Build history of the part. All positions in model axes, mm. Face numbers are marked on the shaded views. A direction names the side the tool comes from. Give positions to 0.01 mm unless a question says otherwise; leave off trailing zeros. Loops run counter-clockwise (first coordinate to the right, second up) from the corner with the lowest first, then second, coordinate; pieces in that order, holes last. Notation, with made-up numbers: M -5,-14 L 35,-14 A17 ccw 35,7 Z; hole C 40.25,-10.75 d8. An arc over 180 degrees is marked long. Put each result on its own line as item: value.
```python
from build123d import *

# Parameters (mm, degrees)
EXTRUDE_1_DEPTH     = 36
EXTRUDE_2_REACH     = 64.61
SKETCH_3_W          = 48
SKETCH_3_H          = 5
CUT_EXTRUDE_3_DEPTH = 63.60990337


with BuildPart() as part:
    # 草圖1 → 伸長1 (new, symmetric)
    with BuildSketch(Plane(origin=(0, 0, 0), x_dir=(0, 0, -1), z_dir=(1, 0, 0))):
        Polygon((0, 0), (40, 0), (40, 32), (30, 32), (10, 8), (0, 8), align=None)
    extrude(amount=EXTRUDE_1_DEPTH, both=True)

    # 伸長2: up to this plane
    extrude_2_end = Plane(origin=(36, 8, -10), z_dir=(0, -0.6401843996644799, -0.7682212795973757))
    # 草圖2 → 伸長2 (add, up to the surface)
    with BuildSketch(Plane.XY, mode=Mode.PRIVATE) as extrude_2_sk1:
        Polygon((28, 8), (-28, 8), (0, 24.165807537), align=None)
    extrude_2_tool1 = split(extrude(extrude_2_sk1.sketch, amount=-EXTRUDE_2_REACH, mode=Mode.PRIVATE), bisect_by=extrude_2_end, keep=Keep.BOTH, mode=Mode.PRIVATE)
    add(extrude_2_tool1.solids().sort_by_distance((0, 13.388603, 0))[0])

    # 草圖3 → 伸長3 (cut, through all)
    with BuildSketch(Plane(origin=(0, 32, 0), x_dir=(1, 0, 0), z_dir=(0, 1, 0))):
        with Locations((0, 37.5)):
            Rectangle(SKETCH_3_W, SKETCH_3_H)
    extrude(amount=-CUT_EXTRUDE_3_DEPTH, mode=Mode.SUBTRACT)


solid = part.part
```
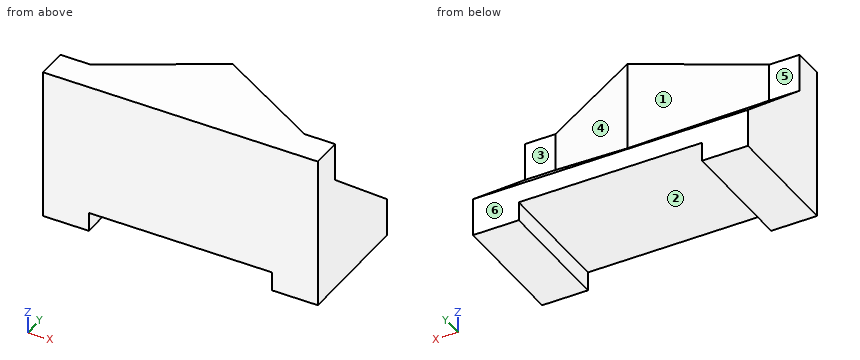
Q1. Slice it at C-C (x = -30.5). List the corners of the cut face in (y, z).
Here are the results:
outline: M 0,-40 L 32,-40 L 32,-30 L 8,-10 L 8,0 L 0,0 Z
Q2. Tool access for the marked faces 4, 5 and 6: list every direction of +Z, -Z, +X, -X, +Y, -Y with a clear straight run to the whole face (end or side of a thin tool).
Here are the results:
face 4: +Z, +X, +Y
face 5: +Z, -X, +Y
face 6: +Z, -Z, +X, -X, +Y
Q3. Slice it at A-A (y = 5). List the corners of the cut face in (x, z), and give its area (3 significant figures).
Here are the results:
outline: M -36,-40 L -24,-40 L -24,-35 L 24,-35 L 24,-40 L 36,-40 L 36,0 L -36,0 Z
area: 2,640 mm²
Q4. Mould opens along X. For the marked faces 1, 2 and 3 say: pulls with the +X half, pulls with the -X half, needs draft (parallel to the pull), parting line crosses it, or undercut.
Here are the results:
face 1: pulls with the -X half
face 2: undercut
face 3: needs draft
Q5. Probe line 1 (Z direction, x = -14, y = 6.5); line 2 (X direction, y = 23.5, z = -11.5); line 3 (Z direction, x = -20, y = 25). List the from-to ranges inside material, lowest first. Write a range as from..to.
Here are the results:
line 1: -35..0
line 2: -1.15..1.15
line 3: -35..-24.17
Q6. Slice it at B-B (z = -6). List the corners of the cut face in (x, y), and give its area (3 significant figures).
Here are the results:
outline: M -36,0 L 36,0 L 36,8 L 28,8 L 0,24.17 L -28,8 L -36,8 Z
area: 1,030 mm²
Q7. Drop flat-ended pins along their axis: pin 1 Ø4 at (x, z) = (31.5, -3) entering from +Y; pin 2 Ø4 at (y, z) = (20, -11.5) entering from -X; pin 3 Ø16 at (x, y) = (4.5, 19) entering from -Z; pin 4 Ø4 at (y, z) = (27.5, -6) entering from -X. Give the stop position or say it passes through.
Here are the results:
pin 1: y = 8
pin 2: x = -10.68
pin 3: z = -35
pin 4: through
Q8. Slice it at D-D (y = 22). List the corners of the cut face in (x, z).
Here are the results:
outline: M -36,-40 L -24,-40 L -24,-35 L 24,-35 L 24,-40 L 36,-40 L 36,-21.67 L 3.75,-21.67 L 3.75,0 L -3.75,0 L -3.75,-21.67 L -36,-21.67 Z
